Part model, mm, in its own coordinate system. Face numbers are marked on the shaded views. A direction names the side the tool comes from. Round coordinates to 2 decimals unless told otherwise and drop trailing zeros. Loops run counter-clockwise (first coordinate to the right, second up) from the corner with the lowest first, then second, coordinate; pieces in that order, holes last.
1) Mould opens along Z. For the marked faces 4, 5 and 6 say: +Z half, -Z half, draft (parallel to the pull), parting line (faces both ways), or undercut.
2) Band-saw the part on A-A, the plane z = 0. Write the cut outline in (x, y) (3 decimals).
3) Band-saw the part on B-B, the plane x = 0. Write the cut outline in (y, z) (3 decimals).
4) Probe line 1 (X direction, y = 80, z = 0); line 2 (X direction, y = 7.25, z = 0) (3 decimals); line 3 (Y direction, x = 27, z = -8). List the from-to ranges inside material, lowest first.
5) Drop flat-ended pins along their axis: P1, Ø2, axis at x = -16.5, y = 54.5, coming from the +Z side; P2, Ø8, axis at y = 33.5, z = -15, coming from the -X side; P3, Ø6, axis at x = -5.5, z = -18.5, coming from the -Y side. Give the stop position or say it passes through.
6) Band-saw the part on D-D, the plane y = 11. Write the cut outline in (x, z) (3 decimals).
7) 3-axis set-ups, long thin cutter, end or side, ignore diameter. For the marked faces 1, 2 and 3: which of +Z, -Z, +X, -X, +Y, -Y reach the whole face in a straight line?
8) Band-saw the part on C-C, the plane y = 65. Write the cut outline in (x, z).
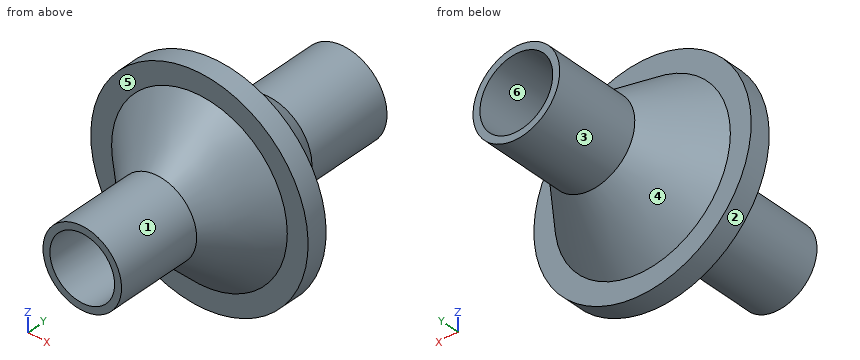
from build123d import *

# Parameters (mm, degrees)
SKETCH1_R           = 11.325
SKETCH1_R_2         = 9.325
BOSS_EXTRUDE1_DEPTH = 25


with BuildPart() as part:
    # Sketch1 → Boss-Extrude1 (new body)
    with BuildSketch(Plane(origin=(0, 0, 0), x_dir=(1, 0, 0), z_dir=(0, 1, 0))):
        with Locations(Location((0, 0, 0), (0, 0, 270))):
            Circle(SKETCH1_R)
        with Locations(Location((0, 0, 0), (0, 0, 270))):
            Circle(SKETCH1_R_2, mode=Mode.SUBTRACT)
    extrude(amount=BOSS_EXTRUDE1_DEPTH)

    # Sketch10 → Revolve1 (revolve)
    with BuildSketch(Plane.XY, mode=Mode.PRIVATE) as revolve1_sk:
        Polygon((-11.325, 25), (-25.325, 39), (-31.325, 39), (-31.325, 42), (-25.325, 42), (-9.325, 25), align=None)
    revolve(revolve1_sk.sketch.rotate(Axis((0, 25, 0), (0, -1, 0)), 270), axis=Axis((0, 25, 0), (0, -1, 0)))

    # Sketch11 → Revolve2 (revolve)
    with BuildSketch(Plane.XY, mode=Mode.PRIVATE) as revolve2_sk:
        Polygon((-31.325, 42), (-31.325, 45), (-25.325, 45), (-12.5, 62), (-12.5, 87), (-10.5, 87), (-10.5, 62), (-25.325, 42), align=None)
    revolve(revolve2_sk.sketch.rotate(Axis((0, 25, 0), (0, -1, 0)), 270), axis=Axis((0, 25, 0), (0, -1, 0)))


solid = part.part
Reported:
1. face 4: parting line
1. face 5: draft
1. face 6: undercut
2. outline: (-31.325, 39) - (-25.325, 39) - (-11.325, 25) - (-11.325, 0) - (-9.325, 0) - (-9.325, 25) - (-25.325, 42) - (-10.5, 62) - (-10.5, 87) - (-12.5, 87) - (-12.5, 62) - (-25.325, 45) - (-31.325, 45) - close; (9.325, 0) - (11.325, 0) - (11.325, 25) - (25.325, 39) - (31.325, 39) - (31.325, 45) - (25.325, 45) - (12.5, 62) - (12.5, 87) - (10.5, 87) - (10.5, 62) - (25.325, 42) - (9.325, 25) - close
3. outline: (0, -11.325) - (25, -11.325) - (39, -25.325) - (39, -31.325) - (45, -31.325) - (45, -25.325) - (62, -12.5) - (87, -12.5) - (87, -10.5) - (62, -10.5) - (42, -25.325) - (25, -9.325) - (0, -9.325) - close; (0, 9.325) - (25, 9.325) - (42, 25.325) - (62, 10.5) - (87, 10.5) - (87, 12.5) - (62, 12.5) - (45, 25.325) - (45, 31.325) - (39, 31.325) - (39, 25.325) - (25, 11.325) - (0, 11.325) - close
4. line 1: x = -12.5 to -10.5, 10.5 to 12.5
4. line 2: x = -11.325 to -9.325, 9.325 to 11.325
4. line 3: y = 39 to 45
5. P1: stops at z = 10
5. P2: stops at x = -19.32
5. P3: stops at y = 29.98
6. outline: circle Ø22.65 at (0, 0); hole circle Ø18.65 at (0, 0)
7. face 1: -Y
7. face 2: +Y, -Y
7. face 3: +Y
8. outline: circle Ø25 at (0, 0); hole circle Ø21 at (0, 0)
